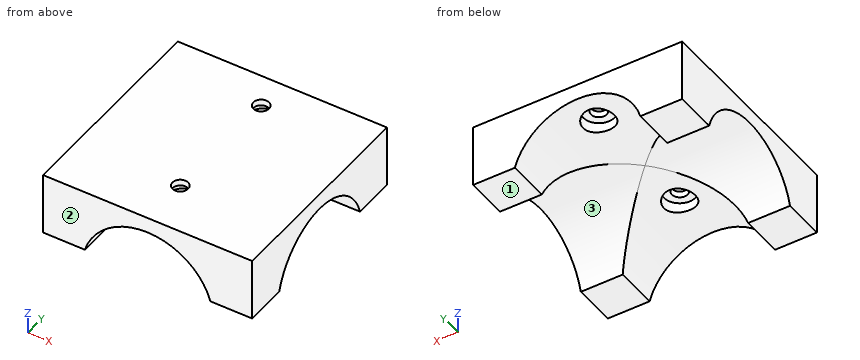
from build123d import *

# Parameters (mm, degrees)
SKETCH1_W           = 40
SKETCH1_H           = 40
BOSS_EXTRUDE1_DEPTH = 12
SKETCH3_R           = 12.5
CUT_EXTRUDE3_DEPTH  = 40
SKETCH11_R          = 12.5
CUT_EXTRUDE4_DEPTH  = 40
SKETCH14_R          = 3
CUT_EXTRUDE7_DEPTH  = 30
SKETCH14_5_R        = 3
SKETCH14_5_R_2      = 1.5
BOSS_EXTRUDE2_DEPTH = 1.2


with BuildPart() as part:
    # Sketch1 → Boss-Extrude1 (new body)
    with BuildSketch(Plane.XY):
        with Locations((-10.055248619, -5.138121547)):
            Rectangle(SKETCH1_W, SKETCH1_H)
    extrude(amount=BOSS_EXTRUDE1_DEPTH)

    # Sketch3 → Cut-Extrude3 (cut)
    with BuildSketch(Plane(origin=(0, 14.861878453, 0), x_dir=(1, 0, 0), z_dir=(0, 1, 0))):
        with Locations((-10.055248619, 3.5)):
            Circle(SKETCH3_R)
    extrude(amount=-CUT_EXTRUDE3_DEPTH, mode=Mode.SUBTRACT)

    # Sketch11 → Cut-Extrude4 (cut)
    with BuildSketch(Plane(origin=(9.944751381, 0, 0), x_dir=(0, 0, -1), z_dir=(1, 0, 0))):
        with Locations((3.5, -5.138121547)):
            Circle(SKETCH11_R)
    extrude(amount=-CUT_EXTRUDE4_DEPTH, mode=Mode.SUBTRACT)

    # Sketch14 → Cut-Extrude7 (cut)
    with BuildSketch(Plane.XY.offset(12)):
        with Locations((-10.055248619, 8.561878453)):
            Circle(SKETCH14_R)
        with Locations((-10.055248619, -15.438121547)):
            Circle(SKETCH14_R)
    extrude(amount=-CUT_EXTRUDE7_DEPTH, mode=Mode.SUBTRACT)

    # Sketch14<5> → Boss-Extrude2 (add)
    # profile 1 of 2: a face of its own
    with BuildSketch(Plane.XY.offset(12)):
        with Locations((-10.055248619, 8.561878453)):
            Circle(SKETCH14_5_R)
        with Locations((-10.055248619, 8.561878453)):
            Circle(SKETCH14_5_R_2, mode=Mode.SUBTRACT)
    # profile 2 of 2: a face of its own
    with BuildSketch(Plane.XY.offset(12)):
        with Locations((-10.055248619, -15.438121547)):
            Circle(SKETCH14_5_R)
        with Locations((-10.055248619, -15.438121547)):
            Circle(SKETCH14_5_R_2, mode=Mode.SUBTRACT)
    extrude(amount=-BOSS_EXTRUDE2_DEPTH)


solid = part.part
Check sheet for the modelled part. Datum: model origin and axes. Units: mm. Face numbers are marked on the shaded views. Round coordinates to 2 decimals unless told otherwise and drop trailing zeros. Order: outer loops, then holes, each group sorted by start corner. A loop starts at its lowest first (then second) coordinate and runs counter-clockwise, first axis right, second up.
Q1. Cross-section at B-B, the plane x = 5. Enter the section's corners in (y, z), plus the area to 3 significant figures.
Filled sheet:
outline: (-25.14, 0) - (-17.14, 0) arc R12.5 cw to (6.86, 0) - (14.86, 0) - (14.86, 12) - (-25.14, 12) - close
area: 321 mm2
Q2. Scan lines: L1, parallel to Z at x = -8, y = 9.5; L2, parallel to Y at x = 1, z = 4.25; L3, parallel to Z at x = -20.5, y = -5. Record each from-to range of solid material in increasing order.
Filled sheet:
L1: z = 10.8 to 12
L2: y = -25.14 to -14.95, 4.67 to 14.86
L3: z = 9 to 12
Q3. Cross-section at A-A, the plane z = 1. Enter the section's corners in (x, y).
Filled sheet:
outline: (-30.06, -25.14) - (-21.72, -25.14) - (-21.72, -16.8) - (-30.06, -16.8) - close; (-30.06, 6.52) - (-21.72, 6.52) - (-21.72, 14.86) - (-30.06, 14.86) - close; (1.61, -25.14) - (9.94, -25.14) - (9.94, -16.8) - (1.61, -16.8) - close; (1.61, 6.52) - (9.94, 6.52) - (9.94, 14.86) - (1.61, 14.86) - close
Q4. Depth check by flat-ended pin: P1, Ø3, axis at x = -11.5, y = 7.5, coming from the -Z side; P2, Ø4, axis at x = -10.06, y = -15.44, coming from the -Z side. Enter the tip coordinate at first touch or a pass-through.
Filled sheet:
P1: stops at z = 8.65
P2: stops at z = 10.8
Q5. Draft check along Y on the marked faces 1, 2 and 3. Enter one of: pulls with the +Y half, pulls with the -Y half, needs draft (parallel to the pull), parting line crosses it, or undercut.
Filled sheet:
face 1: needs draft
face 2: pulls with the -Y half
face 3: undercut
Q6. Cross-section at D-D, the plane y = -7.5. Enter the section's corners in (x, z), plus the area to 3 significant figures.
Filled sheet:
outline: (-30.06, 8.77) - (-12.42, 8.77) arc R12.5 cw to (-7.69, 8.77) - (9.94, 8.77) - (9.94, 12) - (-30.06, 12) - close
area: 128 mm2
Q7. Cross-section at C-C, the plane z = 4.25. Enter the section's corners in (x, y).
Filled sheet:
outline: (-30.06, -25.14) - (-19.86, -25.14) - (-19.86, -14.95) - (-30.06, -14.95) - close; (-30.06, 4.67) - (-19.86, 4.67) - (-19.86, 14.86) - (-30.06, 14.86) - close; (-0.25, -25.14) - (9.94, -25.14) - (9.94, -14.95) - (-0.25, -14.95) - close; (-0.25, 4.67) - (9.94, 4.67) - (9.94, 14.86) - (-0.25, 14.86) - close
